Autodesk Fusion 360 part; units mm, degrees
sketch "Sketch1" plane through (0, 0, 0) normal (0, 1, 0) x (1, 0, 0)
  line L0 (-36, 0) -> (40, 0) construction
  arc A0 (-32, 0) -> (0, -32) centre (0, 0) ccw
  arc A1 (-25.65, 0) -> (0, -25.65) centre (0, 0) ccw
  line L1 (0, -32) -> (0, -25.65)
  line L2 (-25.65, 0) -> (-32, 0)
  dimension "d3" = 25.65
  dimension "d4" = 32
revolve "Revolve1" add sketch "Sketch1" angle 360 about axis through (0, 0, 1.75) along (0, 0, 1)
sketch "Sketch3" plane through (0, 0, 0) normal (0, 0, -1) x (1, 0, 0)
  circle A0 centre (0, 0) radius 32
  circle A1 centre (0, 0) radius 37
  circle A2 centre (0, 0) radius 25.65
  circle A3 centre (0, 0) radius 25.65
  dimension "d10" = 74
extrude "Extrude2" add sketch "Sketch3" against normal blind 5 contours A0 | A1
sketch "Sketch2" plane through (0, 0, 0) normal (0, 0, -1) x (1, 0, 0)
  circle A0 centre (0, 0) radius 28.37
  circle A1 centre (0, 0) radius 32.05
  circle A2 centre (0, 0) radius 37
  circle A3 centre (0, 0) radius 25.65
  dimension "d6" = 56.74
  dimension "d7" = 64.1
extrude "Extrude1" cut sketch "Sketch2" against normal blind 2.794 contours A1
fillet "Fillet1" radius 0.1 2 edges at (-26.4501, 10.259, 2.794) (-29.8811, -11.5898, 2.794)
Build history of the part. All positions in model axes, mm. A direction names the side the tool comes from. Coordinates: 2 decimals unless noted, no trailing zeros. Order: outer loops, then holes, each group sorted by start corner. A loop starts at its lowest first (then second) coordinate and runs counter-clockwise, first axis right, second up. Notation, with made-up numbers: (19.25, -3.5) -> (29.25, -3.5) arc R24 cw to (29.25, 29.5) -> close; hole circle Ø3 at (28.5, 21.25). An arc over 180 degrees is marked (long way). One line per item, written item: value.
(1) Drop flat-ended pins along their axis: pin 1 Ø1.5 at (x, z) = (15.5, 12.5) entering from -Y; pin 2 Ø8 at (y, z) = (15.5, 16) entering from -X; pin 3 Ø1.5 at (y, z) = (9, 5.5) entering from -X; pin 4 Ø3 at (x, y) = (-27, -11) entering from -Z. Give the stop position or say it passes through.
Checked values:
pin 1: y = -25.63
pin 2: x = -26.27
pin 3: x = -36.02
pin 4: z = 0
(2) Probe line 1 (Y direction, x = 0, z = 1); line 2 (X direction, y = 0, z = 0.6); line 3 (Z direction, x = -27, y = 19.5). List the from-to ranges inside material, lowest first. Write a range as [from, to].
Checked values:
line 1: [-37, -32.05], [-28.37, -25.63], [25.63, 28.37], [32.05, 37]
line 2: [-37, -32.05], [-28.37, -25.64], [25.64, 28.37], [32.05, 37]
line 3: [0, 5]
(3) Slice it at A-A, the plane x = 0. List the corners of the cut face in (y, z).
Checked values:
outline: (-37, 0) -> (-32.05, 0) -> (-32.05, 2.69) arc R0.1 cw to (-31.95, 2.79) -> (-28.47, 2.79) arc R0.1 cw to (-28.37, 2.69) -> (-28.37, 0) -> (-25.65, 0) arc R25.65 cw to (25.65, 0) -> (28.37, 0) -> (28.37, 2.69) arc R0.1 cw to (28.47, 2.79) -> (31.95, 2.79) arc R0.1 cw to (32.05, 2.69) -> (32.05, 0) -> (37, 0) -> (37, 5) -> (31.61, 5) arc R32 ccw to (-31.61, 5) -> (-37, 5) -> close
(4) Mould opens along X. For faces 4 (the cylindrical face through (-25.434, 19.502, 1.328)), 5 (the flat face through (21, 15, 0)), 6 (the cylindrical face through (-8.02, 36.12, 2.46)) say: pulls with the +X half, pulls with the -X half, needs draft (parallel to the pull), parting line crosses it, or undercut.
Checked values:
face 4: undercut
face 5: needs draft
face 6: parting line crosses it
(5) Slice it at C-C, the plane z = 11. List the corners of the cut face in (x, y), plus the area to 3 significant figures.
Checked values:
outline: circle Ø60.1 at (0, 0); hole circle Ø46.34 at (0, 0)
area: 1,150 mm2
(6) Slice it at D-D, the plane z = 30. List the corners of the cut face in (x, y).
Checked values:
outline: circle Ø22.27 at (0, 0)
(7) Tool access for faces 1 (the flat face through (11.1, -30.3, 0)), 2 (the cylindrical face through (26.207, 10.866, 1.328)), 3 (the flat face through (27, -17, 5)): list every direction of +Z, -Z, +X, -X, +Y, -Y with a clear straight run to the whole face (end or side of a thin tool).
Checked values:
face 1: -Z, +X, -X, +Y, -Y
face 2: -Z
face 3: +Z
